Verification items for the finished model (mm, model axes). Face numbers are marked on the shaded views. A direction names the side the tool comes from. Round coordinates to 2 decimals unless told otherwise and drop trailing zeros. Put each result on its own line as item: value.
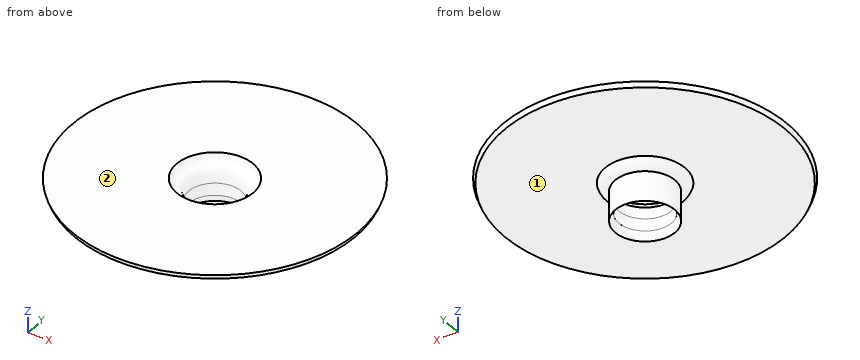
```python
from build123d import *


with BuildPart() as f1:
    # F0 (on Front) → F1 (revolve)
    with BuildSketch(Plane.XZ):
        with BuildLine():
            ThreePointArc((39.6875, -11.2468861043), (48.1489607267, -7.6980115894), (53.1421005726, 0))
            Line((53.1421005726, 0), (186.69, 0))
            Line((186.69, 0), (189.23, 6.35))
            Line((189.23, 6.35), (50.8, 6.35))
            add(Edge.make_bspline(
                [(50.8, 6.35), (49.1728301439, -4.4232065161), (36.2611646426, -1.9466716062), (34.8222671813, -16.0190971942), (34.925, -23.8922853023)],
                knots=[0, 0, 0, 0, 0.4885222498, 1, 1, 1, 1], degree=3))
            Line((34.925, -23.8922853023), (34.925, -40.0551594794))
            add(Edge.make_bspline(
                [(39.6875, -50.8), (38.2820304334, -45.8264946938), (34.8677070156, -44.9470542371), (34.925, -40.0551594794)],
                knots=[0, 0, 0, 0, 11.75299979, 11.75299979, 11.75299979, 11.75299979], degree=3))
            Line((39.6875, -50.8), (39.6875, -11.2468861043))
        make_face()
    revolve(axis=Axis((0, 0, 2.4035767974), (0, 0, -1)))


solid = f1.part
```
Item 1: Depth check by flat-ended pin: pin 1 Ø1 at (y, z) = (31, -8) entering from -X; pin 2 Ø1.5 at (x, z) = (40.5, -2) entering from -Y. Enter the tip coordinate at first touch or a pass-through.
Geometry check:
pin 1: x = -37.25
pin 2: y = -34.31
Item 2: Tool access check on the marked faces 1 and 2. Record the directions out of +Z, -Z, +X, -X, +Y, -Y that give a thin tool (end or side, any length) a straight path to the whole face; none if there is none.
Geometry check:
face 1: -Z
face 2: +Z, +X, -X, +Y, -Y
Item 3: Material ranges on line 1 along Y through (x, z) = (0, -28) (1 decimal); line 2 along Z through (x, y) = (-71.5, 77), recorded low to high.
Geometry check:
line 1: -39.7 to -34.9, 34.9 to 39.7
line 2: 0 to 6.35
